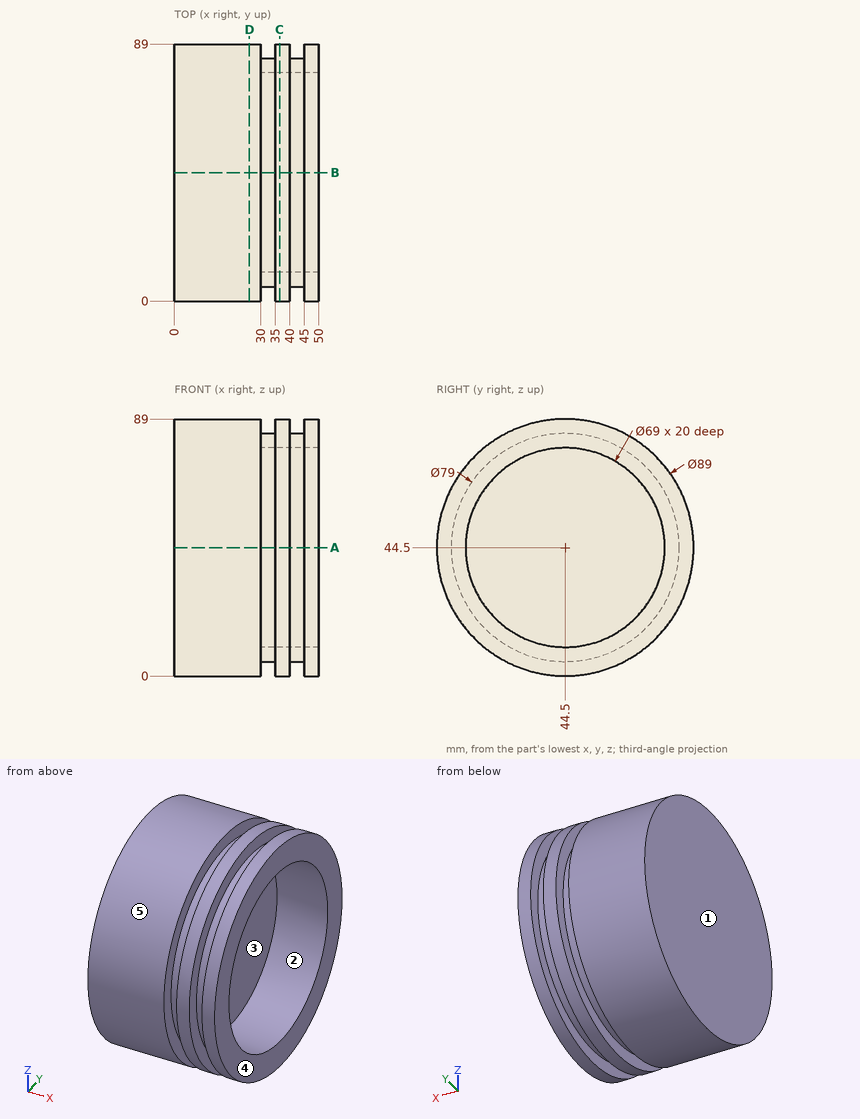
Here's the drawing with two shaded views (mm, measured from the low corner). I have some questions. A direction names the side the tool comes from. Coordinates: 2 decimals unless noted, no trailing zeros. Write each loop counter-clockwise with the first axis right and the second up, starting at its lowest first coordinate (ties: lowest second). Pieces come first, ordered by that corner, then holes.
Item 1: On a 3-axis mill with a long thin cutter (end or side, diameter ignored), from which of +Z, -Z, +X, -X, +Y, -Y can I reach the whole of each face in a straight line? I mean the marked faces 1 and 2. Say none if no direction works.
Item 2: Will these pins go through, and if not, where does the flat tip stop? pin 1 (8 mm diameter, centred on x = 12, y = 36.5, fed in from +Z); pin 2 (8 mm diameter, centred on y = 41.5, z = 61.5, fed in from +X); pin 3 (1.5 mm diameter, centred on x = 19, y = 40.5, fed in from +Z).
Item 3: If we mould it in two halves opening along Y, with no side actions, what happens to the marked faces 3, 4 and 5? For each: +Y half, -Y half, draft (parallel to the pull), parting line (faces both ways), or undercut.
Item 4: If I drill on line 1 (Z direction, x = 36.5, y = 44.5); line 2 (Z direction, x = 43, y = 44), over which ranges is the centre line in solid material (lowest first)?
Item 5: I want a section at D-D on x = 26. Write out the boundary of the cut face in (y, z), and give its area (3 significant figures).
Item 6: I want a section at A-A on z = 44.5. Write out the boundary of the cut face in (x, y), and give its area (3 significant figures).
Item 7: I want a section at C-C on x = 36.5. Write out the boundary of the cut face in (y, z), and give its area (3 significant figures).
Findings below:
1. face 1: +Z, -Z, -X, +Y, -Y
1. face 2: +X
2. pin 1: stops at z = 88.82
2. pin 2: stops at x = 30
2. pin 3: stops at z = 88.88
3. face 3: undercut
3. face 4: draft
3. face 5: parting line
4. line 1: z = 0 to 10, 79 to 89
4. line 2: z = 5 to 10, 79 to 84
5. outline: circle Ø89 at (44.5, 44.5)
5. area: 6,220 mm2
6. outline: (0, 0) - (30, 0) - (30, 5) - (35, 5) - (35, 0) - (40, 0) - (40, 5) - (45, 5) - (45, 0) - (50, 0) - (50, 10) - (30, 10) - (30, 79) - (50, 79) - (50, 89) - (45, 89) - (45, 84) - (40, 84) - (40, 89) - (35, 89) - (35, 84) - (30, 84) - (30, 89) - (0, 89) - close
6. area: 2,970 mm2
7. outline: circle Ø89 at (44.5, 44.5); hole circle Ø69 at (44.5, 44.5)
7. area: 2,480 mm2
